Drawing for the job (mm, zero at the part's lowest x, y, z). A direction names the side the tool comes from. Give positions to 0.01 mm unless a question says otherwise; leave off trailing zeros. Write each loop counter-clockwise with the first axis right and the second up, starting at its lowest first coordinate (ties: lowest second). Pieces come first, ordered by that corner, then holes. Notation, with made-up numbers: (-36.5, 0) - (22.5, 0) arc R8 ccw to (22.5, 13) - close; hole circle Ø2 at (82, -24.75). An arc over 180 degrees is marked (long way). Use CSV: the item, a comma, the result in double quotes.
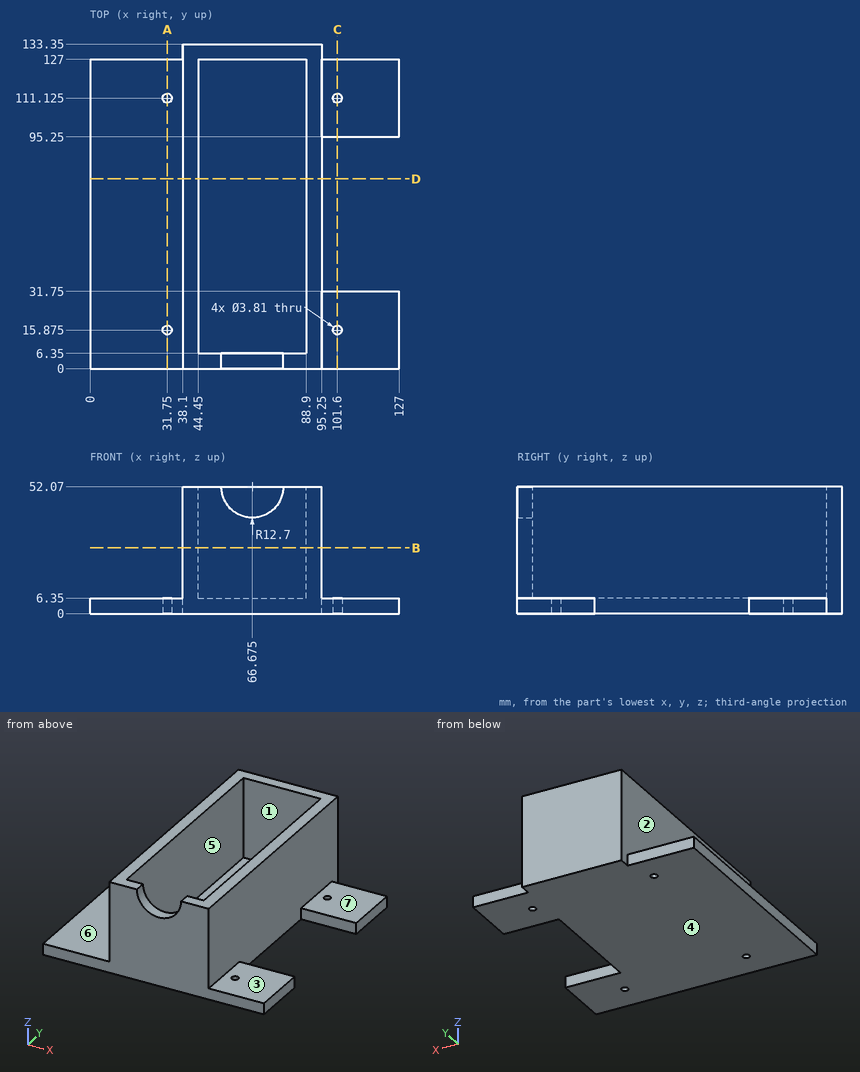
(1) 3-axis set-ups, long thin cutter, end or side, ignore diameter. For the marked faces 4, 5, 6 and 7: which of +Z, -Z, +X, -X, +Y, -Y reach the whole face in a straight line?
Checked values:
face 4,"-Z, +X, -X, +Y, -Y"
face 5,"+Z"
face 6,"+Z, -X, +Y, -Y"
face 7,"+Z, +X, +Y, -Y"
(2) Saw through at B-B, the plane z = 27. List the corners of the cut face in (x, y), then the cut area to 3 significant figures.
Checked values:
outline,"(38.1, 0) - (95.25, 0) - (95.25, 133.35) - (38.1, 133.35) - close; hole (44.45, 6.35) - (88.9, 6.35) - (88.9, 127) - (44.45, 127) - close"
area,"2,260 mm^2"
(3) Saw through at D-D, the plane y = 78. List the corners of the cut face in (x, z), then the cut area to 3 significant figures.
Checked values:
outline,"(0, 0) - (95.25, 0) - (95.25, 52.07) - (88.9, 52.07) - (88.9, 6.35) - (44.45, 6.35) - (44.45, 52.07) - (38.1, 52.07) - (38.1, 6.35) - (0, 6.35) - close"
area,"1,190 mm^2"
(4) Saw through at C-C, the plane x = 101.6. List the corners of the cut face in (y, z).
Checked values:
outline,"(0, 0) - (13.97, 0) - (13.97, 6.35) - (0, 6.35) - close; (17.78, 0) - (31.75, 0) - (31.75, 6.35) - (17.78, 6.35) - close; (95.25, 0) - (109.22, 0) - (109.22, 6.35) - (95.25, 6.35) - close; (113.03, 0) - (127, 0) - (127, 6.35) - (113.03, 6.35) - close"
(5) Saw through at A-A, the plane x = 31.75. List the corners of the cut face in (y, z).
Checked values:
outline,"(0, 0) - (13.97, 0) - (13.97, 6.35) - (0, 6.35) - close; (17.78, 0) - (109.22, 0) - (109.22, 6.35) - (17.78, 6.35) - close; (113.03, 0) - (127, 0) - (127, 6.35) - (113.03, 6.35) - close"
(6) Pull direction X, two halves, no side cores. Call the marked faces 1, 2 and 3: released by +X, released by -X, zero draft, split by the parting line, or undercut.
Checked values:
face 1,"undercut"
face 2,"released by -X"
face 3,"zero draft"
(7) Wall check: probe 1 along Y at (x, z) = (31.75, 3.5); probe 2 along Y at (x, z) = (101.6, 4); probe 3 along Y at (x, z) = (45, 48.5). Give the ranges that are in metal, low to high. Write a range as [from, to].
Checked values:
probe 1,"y = [0, 13.97], [17.78, 109.22], [113.03, 127]"
probe 2,"y = [0, 13.97], [17.78, 31.75], [95.25, 109.22], [113.03, 127]"
probe 3,"y = [0, 6.35], [127, 133.35]"
(8) Flat gauge pins, fed straight in: P1, Ø6, axis at y = 70, z = 26.5, coming from the -X side; P2, Ø9.5, axis at x = 106.5, y = 10, coming from the +Z side; P3, Ø3, axis at x = 117.5, z = 4, coming from the +Y side. Where does each tip first touch, or does it go through?
Checked values:
P1,"stops at x = 38.1"
P2,"stops at z = 6.35"
P3,"stops at y = 127"
